```python
from build123d import *

# Parameters (mm, degrees)
SKETCH1_W           = 228.6
SKETCH1_H           = 101.6
BOSS_EXTRUDE1_DEPTH = 2.54
CUT_EXTRUDE1_REACH  = 4.54
SKETCH2_R           = 3.175


with BuildPart() as part:
    # Sketch1 → Boss-Extrude1 (new body)
    with BuildSketch(Plane(origin=(0, 0, 0), x_dir=(0, 0, -1), z_dir=(1, 0, 0))):
        Rectangle(SKETCH1_W, SKETCH1_H)
    extrude(amount=-BOSS_EXTRUDE1_DEPTH)

    # Sketch2 → Cut-Extrude1 (cut, up to next)
    with BuildSketch(Plane(origin=(0, 0, 0), x_dir=(0, 0, -1), z_dir=(1, 0, 0)), mode=Mode.PRIVATE) as cut_extrude1_sk1:
        with Locations((-101.6, 0)):
            Circle(SKETCH2_R)
    cut_extrude1_tool1 = extrude(cut_extrude1_sk1.sketch, amount=-CUT_EXTRUDE1_REACH, mode=Mode.PRIVATE) & part.part
    add(cut_extrude1_tool1.solids().sort_by_distance((0, 0, 101.6))[0], mode=Mode.SUBTRACT)


solid = part.part
```
Here's how the part is built. I have some questions about the finished solid (model axes, mm). Coordinates: 2 decimals unless noted, no trailing zeros. Order: outer loops, then holes, each group sorted by start corner. A loop starts at its lowest first (then second) coordinate and runs counter-clockwise, first axis right, second up.
1) Will this pin go through, and if not, where does the flat tip stop? pin 1 (10 mm diameter, centred on y = 0, z = 101.6, fed in from -X).
2) Imagine slicing it at A-A on y = 0. List the corners of the cut face in (x, z) for me (3 decimals).
3) Imagine slicing it at B-B on z = 101.6. List the corners of the cut face in (x, y) for me (3 decimals).
4) We'd pull the mould along Y, two halves only. Please class faces 1 (the face through (-1.25, 0.14, 104.77)), 2 (the face through (-2.54, 1, 2)): +Y half, -Y half, draft (parallel to the pull), parting line (faces both ways), or undercut.
5) I need wall thicknesses on line 1 (Y direction, x = -0.85, z = 101.6) (3 decimals); line 2 (Y direction, x = -0.95, z = 99). Which ranges of each line are inside material? Lowest first, please.
Response values:
1. pin 1: stops at x = -2.54
2. outline: (-2.54, -114.3) - (0, -114.3) - (0, 98.425) - (-2.54, 98.425) - close; (-2.54, 104.775) - (0, 104.775) - (0, 114.3) - (-2.54, 114.3) - close
3. outline: (-2.54, -50.8) - (0, -50.8) - (0, -3.175) - (-2.54, -3.175) - close; (-2.54, 3.175) - (0, 3.175) - (0, 50.8) - (-2.54, 50.8) - close
4. face 1: undercut
4. face 2: draft
5. line 1: y = -50.8 to -3.175, 3.175 to 50.8
5. line 2: y = -50.8 to -1.82, 1.82 to 50.8
